Check sheet for the drawn part. Datum: minimum x, y, z corner. Units: mm. A direction names the side the tool comes from. Give positions to 0.01 mm unless a question says otherwise; leave off trailing zeros. Write each loop counter-clockwise with the first axis right and the second up, starting at its lowest first coordinate (ties: lowest second). Pieces come first, ordered by that corner, then holes. Notation, with made-up numbers: (38.5, -6.5) - (63.5, -6.5) arc R27 ccw to (63.5, 23.5) - close; hole circle Ø2 at (-1.75, 4.25). An arc over 180 degrees is marked (long way). One line per question, with ' | ' between items. Start each with the question number.
Q1. Release check for a two-part mould opening along X. For the marked faces 1, 2 and 3 record: +X half, -X half, draft (parallel to the pull), parting line (faces both ways), or undercut.
Q2. Set-up check for the marked faces 4 and 5: record each of +Z, -Z, +X, -X, +Y, -Y from which the full face is reachable in a straight line by a thin tool's end or side.
Q3. Thickness scan on L1, parallel to Z at x = 34, y = 8; L2, parallel to X at y = 10.5, z = 3; L3, parallel to X at y = 3, z = 3.75. Record the ranges inside material, lowest first. Write a range as [from, to].
Q4. Gauge pin test, flat ends, axial feed: P1, Ø2, axis at y = 8, z = 5.5, coming from the -X side; P2, Ø1, axis at x = 29.5, z = 6, coming from the +Y side; P3, Ø1.2, axis at x = 4.5, z = 5, coming from the -Y side; P4, Ø1.5, axis at x = 29.5, z = 7, coming from the +Y side. Record the tip position at first contact, or that the pin passes through.
Q5. Section check A-A on z = 4. Record the boundary of the cut face in (x, y).
Q6. Section check C-C on y = 3.5. Record the boundary of the cut face in (x, z), and give its area (3 significant figures).
Q7. Section check B-B on x = 19. Record the boundary of the cut face in (y, z), and give its area (3 significant figures).
Q8. Section check D-D on x = 10. Record the boundary of the cut face in (y, z).
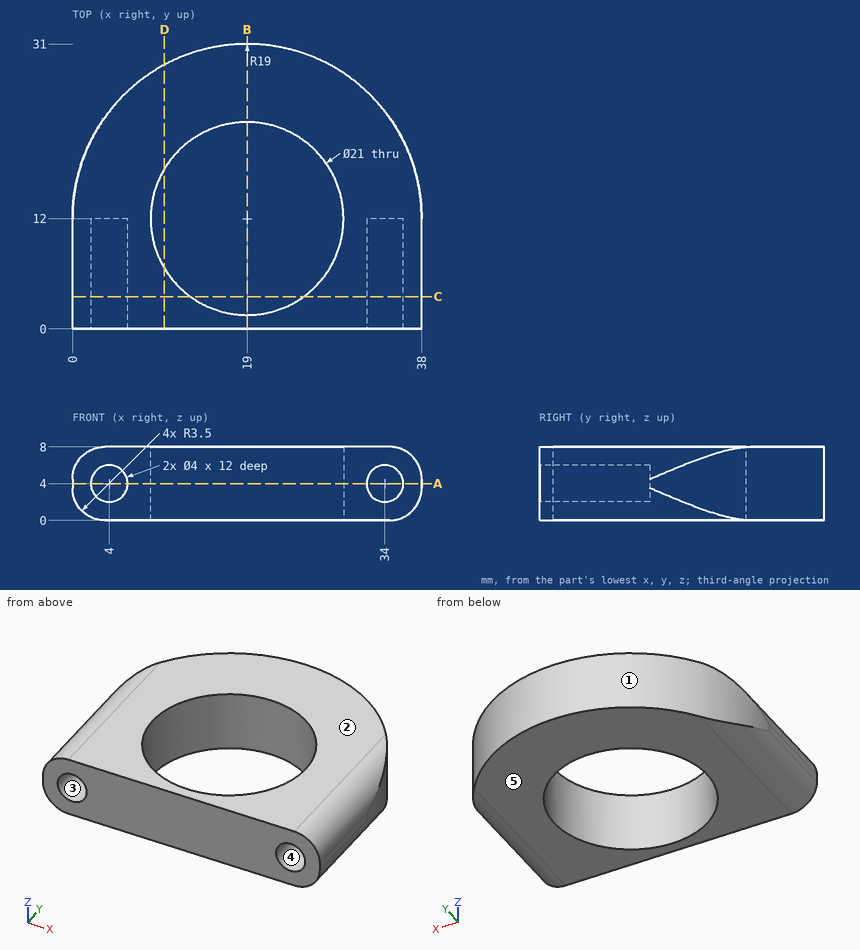
Working result:
1) face 1: parting line | face 2: draft | face 3: undercut
2) face 4: -Y | face 5: -Z, +X, -X, +Y, -Y
3) L1: z = [0, 2], [6, 8] | L2: x = [0.04, 2.27], [5.73, 8.61], [29.39, 32.27], [35.73, 37.96] | L3: x = [0, 2.02], [5.98, 13.59], [24.41, 32.02], [35.98, 38]
4) P1: stops at x = 0 | P2: stops at y = 28.16 | P3: stops at y = 12 | P4: stops at y = 28.31
5) outline: (0, 0) - (2, 0) - (2, 12) - (6, 12) - (6, 0) - (32, 0) - (32, 12) - (36, 12) - (36, 0) - (38, 0) - (38, 12) arc R19 ccw to (0, 12) - close; hole circle Ø21 at (19, 12)
6) outline: (0, 3.5) arc R3.5 ccw to (3.5, 0) - (12.84, 0) - (12.84, 8) - (3.5, 8) arc R3.5 ccw to (0, 4.5) - close; (25.16, 0) - (34.5, 0) arc R3.5 ccw to (38, 3.5) - (38, 4.5) arc R3.5 ccw to (34.5, 8) - (25.16, 8) - close; hole circle Ø4 at (4, 4); hole circle Ø4 at (34, 4) | area: 170 mm2
7) outline: (0, 0) - (1.5, 0) - (1.5, 8) - (0, 8) - close; (22.5, 0) - (31, 0) - (31, 8) - (22.5, 8) - close | area: 80.0 mm2
8) outline: (0, 0) - (6.59, 0) - (6.59, 8) - (0, 8) - close; (17.41, 0) - (28.73, 0) - (28.73, 8) - (17.41, 8) - close
